```python
from build123d import *

# Parameters (mm, degrees)
SKETCH2_W                = 12
SKETCH2_H                = 4
BOSS_EXTRUDE2_DEPTH      = 20
SKETCH4_R                = 45
BOSS_EXTRUDE3_DEPTH      = 4.5
FILLET1_R                = 4
CUT_EXTRUDE1_REACH       = 100.393
SKETCH5_R                = 3
FILLET2_R                = 4
CIRPATTERN5_COUNT        = 3
FILLET1_OF_CIRPATTERN5_R = 4
FILLET2_OF_CIRPATTERN5_R = 4
CAVITY1_START            = 21
CAVITY1_DEPTH            = 3.5
CAVITY2_START            = 21
CAVITY2_DEPTH            = 3.5


# Read off the part's stored shape, not the designer's step: Cavity1, Cavity2
with BuildPart() as part:
    # Sketch2 → Boss-Extrude2 (new body)
    with BuildSketch(Plane(origin=(0, 0, 0), x_dir=(1, 0, 0), z_dir=(0, 1, 0))):
        with Locations((0, 30.848076211)):
            Rectangle(SKETCH2_W, SKETCH2_H)
    boss_extrude2 = extrude(amount=BOSS_EXTRUDE2_DEPTH)

    # Sketch4 → Boss-Extrude3 (add)
    with BuildSketch(Plane(origin=(0, 20, 0), x_dir=(1, 0, 0), z_dir=(0, 1, 0))):
        with Locations(Location((0, -6.151923789, 0), (0, 0, 270))):
            Circle(SKETCH4_R)
    extrude(amount=BOSS_EXTRUDE3_DEPTH)

    # Fillet1
    fillet1_edges = [part.edges().sort_by_distance(p)[0] for p in [
        (-6, 20, -30.848076211),
        (6, 20, -30.848076211),
        (0, 20, -32.848076211),
    ]]
    fillet(fillet1_edges, radius=FILLET1_R)

    # Sketch5 → Cut-Extrude1 (cut, up to next)
    with BuildSketch(Plane(origin=(0, 0, -32.848076211), x_dir=(-1, 0, 0), z_dir=(0, 0, -1)), mode=Mode.PRIVATE) as cut_extrude1_sk1:
        with Locations((0, 6)):
            Circle(SKETCH5_R)
    cut_extrude1_tool1 = extrude(cut_extrude1_sk1.sketch, amount=-CUT_EXTRUDE1_REACH, mode=Mode.PRIVATE) & part.part
    cut_extrude1 = cut_extrude1_tool1.solids().sort_by_distance((0, 6, -32.848076))[0]
    add(cut_extrude1, mode=Mode.SUBTRACT)

    # Fillet2
    fillet2_edges = [part.edges().sort_by_distance(p)[0] for p in [
        (-6, 0, -30.848076211),
        (6, 0, -30.848076211),
    ]]
    fillet(fillet2_edges, radius=FILLET2_R)

    # CirPattern5: Boss-Extrude2, Cut-Extrude1 ×3 about axis
    cirpattern5_axis = Axis((0, 0, 6.151923789), (0, 1, 0))
    add([boss_extrude2.rotate(cirpattern5_axis, i * 360 / CIRPATTERN5_COUNT) for i in range(1, CIRPATTERN5_COUNT)])
    add([cut_extrude1.rotate(cirpattern5_axis, i * 360 / CIRPATTERN5_COUNT) for i in range(1, CIRPATTERN5_COUNT)], mode=Mode.SUBTRACT)

    # Fillet1 of CirPattern5
    fillet1_of_cirpattern5_edges = [part.edges().sort_by_distance(p)[0] for p in [
        (-29.04293994, 20, 29.848076211),
        (-35.04293994, 20, 19.455771366),
        (-33.774990748, 20, 25.651923789),
        (35.04293994, 20, 19.455771366),
        (29.04293994, 20, 29.848076211),
        (33.774990748, 20, 25.651923789),
    ]]
    fillet(fillet1_of_cirpattern5_edges, radius=FILLET1_OF_CIRPATTERN5_R)

    # Fillet2 of CirPattern5
    fillet2_of_cirpattern5_edges = [part.edges().sort_by_distance(p)[0] for p in [
        (-29.04293994, 0, 29.848076211),
        (-35.04293994, 0, 19.455771366),
        (35.04293994, 0, 19.455771366),
        (29.04293994, 0, 29.848076211),
    ]]
    fillet(fillet2_of_cirpattern5_edges, radius=FILLET2_OF_CIRPATTERN5_R)

    # Cavity1 outline → Cavity1 (cut)
    with BuildSketch(Plane(origin=(0, 0, 0), x_dir=(1, 0, 0), z_dir=(0, 1, 0)).offset(CAVITY1_START)):
        with BuildLine():
            ThreePointArc((2.442725539, -10.067144534), (1.841235151, -9.627440673), (1.102669127, -9.725677123))
            ThreePointArc((1.102669127, -9.725677123), (-28.135128354, -2.275427339), (-21.973365635, 27.260782702))
            ThreePointArc((-21.973365635, 27.260782702), (-21.560444182, 27.88096497), (-21.690953471, 28.614516261))
            ThreePointArc((-21.690953471, 28.614516261), (-22.33514846, 29.064110473), (-23.10537251, 28.909588462))
            ThreePointArc((-23.10537251, 28.909588462), (-29.831959556, -3.334088698), (2.085950749, -11.467273303))
            ThreePointArc((2.085950749, -11.467273303), (2.563344478, -10.843400426), (2.442725539, -10.067144534))
        make_face()
    extrude(amount=CAVITY1_DEPTH, mode=Mode.SUBTRACT)

    # Cavity2 outline → Cavity2 (cut)
    with BuildSketch(Plane(origin=(0, 0, 0), x_dir=(1, 0, 0), z_dir=(0, 1, 0)).offset(CAVITY2_START)):
        with BuildLine():
            ThreePointArc((-2.442725539, -2.236703043), (-1.841235151, -2.676406904), (-1.102669127, -2.578170454))
            ThreePointArc((-1.102669127, -2.578170454), (28.135128354, -10.028420238), (21.973365635, -39.564630279))
            ThreePointArc((21.973365635, -39.564630279), (21.560444182, -40.184812547), (21.690953471, -40.918363839))
            ThreePointArc((21.690953471, -40.918363839), (22.33514846, -41.36795805), (23.10537251, -41.213436039))
            ThreePointArc((23.10537251, -41.213436039), (29.831959556, -8.96975888), (-2.085950749, -0.836574274))
            ThreePointArc((-2.085950749, -0.836574274), (-2.563344478, -1.460447151), (-2.442725539, -2.236703043))
        make_face()
    extrude(amount=CAVITY2_DEPTH, mode=Mode.SUBTRACT)


solid = part.part
```
Source: CAD feature listing. Evaluate the final solid. Frame: model axes, mm. A direction names the side the tool comes from. Give positions to 0.01 mm unless a question says otherwise; leave off trailing zeros. Write each loop counter-clockwise with the first axis right and the second up, starting at its lowest first coordinate (ties: lowest second). Pieces come first, ordered by that corner, then holes.
1. Section query D-D (z = 6.5). Return the cut outline in (x, y), then the cut area to 3 significant figures.
2. First-contact query: pin 1 (3 mm diameter, centred on y = 12.5, z = -31.5, fed in from +X); pin 2 (1.5 mm diameter, centred on x = -12.5, y = 17.5, fed in from -Z); pin 3 (2 mm diameter, centred on x = 7, z = -0.5, fed in from -Y); pin 4 (13 mm diameter, centred on x = 1, y = 8.5, fed in from -Z). Flat tips, straight axial feed; report the tip coordinate or a pass-through.
3. Section query A-A (y = 11.75). Return the cut outline in (x, z) (3 decimals).
4. Material intervals for line 1 along Y through (x, z) = (0, -31.5); line 2 along Y through (x, z) = (-4.5, 25); line 3 along X through (y, z) = (18.25, 22.5), sorted ascending.
5. Section query C-C (y = 6). Return the cut outline in (x, z) (3 decimals), then the cut area to 3 significant figures.
6. Pull-direction query (Z, two-part tool) for faces 6 (the face through (34.5, 1.2, 20.46)), 7 (the face through (-32.39, 3.07, 24.1)), 8 (the face through (1, 24.5, 6)); classes: +Z half, -Z half, draft (parallel to the pull), parting line (faces both ways), or undercut.
7. Section query B-B (x = 0). Return the cut outline in (y, z), then the cut area to 3 significant figures.
8. Access query for faces 1 (the face through (6, 10, -31)), 2 (the face through (-30.241, 9.86, 23.773)), 3 (the face through (-29.183, 19.302, 31.94)), 4 (the face through (33.817, 9.666, 25.579)), 5 (the face through (1, 20, 6)). Directions: +Z, -Z, +X, -X, +Y, -Y. A direction counts if a zero-diameter tool reaches every point of the face in a straight line with its end or side. Return the directions, or none.
Output values:
1. outline: (-45, 20) - (45, 20) - (45, 24.5) - (28.06, 24.5) - (28.06, 21) - (25.39, 21) - (25.39, 24.5) - (-24.7, 24.5) - (-24.7, 21) - (-27.47, 21) - (-27.47, 24.5) - (-45, 24.5) - close
1. area: 386 mm2
2. pin 1: stops at x = 6
2. pin 2: passes through
2. pin 3: stops at y = 20
2. pin 4: stops at z = -32.85
3. outline: (-36.775, 20.456) - (-33.311, 18.456) - (-27.311, 28.848) - (-30.775, 30.848) - close; (-6, -32.848) - (6, -32.848) - (6, -28.848) - (-6, -28.848) - close; (27.311, 28.848) - (33.311, 18.456) - (36.775, 20.456) - (30.775, 30.848) - close
4. line 1: y = 0 to 3, 9 to 24.5
4. line 2: y = 20 to 24.5
4. line 3: x = -36.39 to -30.98, 30.98 to 36.39
5. outline: (-36.775, 20.456) - (-33.311, 18.456) - (-31.811, 21.054) - (-35.275, 23.054) - close; (-32.275, 28.25) - (-28.811, 26.25) - (-27.311, 28.848) - (-30.775, 30.848) - close; (-6, -32.848) - (-3, -32.848) - (-3, -28.848) - (-6, -28.848) - close; (3, -32.848) - (6, -32.848) - (6, -28.848) - (3, -28.848) - close; (27.311, 28.848) - (28.811, 26.25) - (32.275, 28.25) - (30.775, 30.848) - close; (31.811, 21.054) - (33.311, 18.456) - (36.775, 20.456) - (35.275, 23.054) - close
5. area: 72.0 mm2
6. face 6: -Z half
6. face 7: undercut
6. face 8: draft
7. outline: (0, -32.85) - (3, -32.85) - (3, -28.85) - (0, -28.85) - close; (9, -32.85) - (16, -32.85) arc R4 cw to (20, -36.85) - (20, -38.85) - (24.5, -38.85) - (24.5, -0.21) - (21, -0.21) - (21, 2) - (24.5, 2) - (24.5, 10.31) - (21, 10.31) - (21, 12.51) - (24.5, 12.51) - (24.5, 51.15) - (20, 51.15) - (20, -28.85) - (9, -28.85) - close
7. area: 449 mm2
8. face 1: +Z, -Z, +X, -Y
8. face 2: -Z, -Y
8. face 3: +Z, -Y
8. face 4: +Z, +X, -Y
8. face 5: -Y
